Geometry check sheet. Reference: the model listing, model coordinates, mm. A direction names the side the tool comes from. Round coordinates to 2 decimals unless told otherwise and drop trailing zeros. Write each loop counter-clockwise with the first axis right and the second up, starting at its lowest first coordinate (ties: lowest second). Pieces come first, ordered by that corner, then holes. Notation, with made-up numbers: (39.25, 29) - (67.25, 29) arc R33 cw to (67.25, 64) - close; hole circle Ø6 at (20.5, -15.75). An arc over 180 degrees is marked (long way). Return JSON: item names as keys, results as strings.
```python
from build123d import *

# Parameters (mm, degrees)
PAD008_DEPTH = 30
SKETCH003_W  = 24.676034
SKETCH003_H  = 10
PAD002_DEPTH = 25
PAD001_DEPTH = 20
SKETCH002_R  = 5.5
POCKET_DEPTH = 24
PAD007_DEPTH = 40
PAD_DEPTH    = 40


with BuildPart() as pad008:
    # Sketch009 → Pad008 (new body)
    with BuildSketch(Plane.YZ.offset(-17)):
        with BuildLine():
            ThreePointArc((10.172884, 61.128702), (0, 71.301585), (-10.172884, 61.128702))
            Line((-10.172884, 61.128702), (-10.172884, 11.128702))
            ThreePointArc((-10.172884, 11.128702), (0, 0.955818), (10.172884, 11.128702))
            Line((10.172884, 61.128702), (10.172884, 11.128702))
        make_face()
    extrude(amount=PAD008_DEPTH)


with BuildPart() as pad002:
    # Sketch003 → Pad002 (new body)
    with BuildSketch(Plane(origin=(10, 0, 1), x_dir=(1, 0, 0), z_dir=(0, 0, 1))):
        with Locations((25.629245, 0)):
            Rectangle(SKETCH003_W, SKETCH003_H)
    extrude(amount=PAD002_DEPTH)


with BuildPart() as cut:
    # Sketch001 → Pad001 (new body)
    with BuildSketch(Plane(origin=(10, 10, 0), x_dir=(1, 0, 0), z_dir=(0, -1, 0))):
        with BuildLine():
            ThreePointArc((23.375231, 20.790424), (13.375231, 10.790424), (23.375231, 0.790424))
            Line((23.375231, 0.790424), (27.963482, 0.790424))
            ThreePointArc((27.963482, 0.790424), (37.963482, 10.790424), (27.963482, 20.790424))
            Line((23.375231, 20.790424), (27.963482, 20.790424))
        make_face()
    extrude(amount=PAD001_DEPTH)

    # Sketch002 → Pocket (cut)
    with BuildSketch(Plane(origin=(10, -10, 0), x_dir=(1, 0, 0), z_dir=(0, -1, 0))):
        with Locations((25.214981, 10.647934)):
            Circle(SKETCH002_R)
    extrude(amount=-POCKET_DEPTH, mode=Mode.SUBTRACT)

    # Cut: cut Pad002
    add(pad002.part, mode=Mode.SUBTRACT)


with BuildPart() as pad007:
    # Sketch008 → Pad007 (new body)
    with BuildSketch(Plane.XZ.offset(-20)):
        with BuildLine():
            ThreePointArc((11.056906, 25.953392), (1.290425, 15.054425), (-2.307496, 0.868989))
            ThreePointArc((1.093916, 25.953392), (-3.737473, 13.835707), (-2.307496, 0.868989))
            Line((1.093916, 25.953392), (11.056906, 25.953392))
        make_face()
    extrude(amount=PAD007_DEPTH)


with BuildPart() as cut001:
    # Sketch → Pad (new body)
    with BuildSketch(Plane.XZ.offset(-20)):
        with BuildLine():
            Line((-4.143037, -1.678632), (67.891418, -1.678632))
            Line((63.009144, 0.821368), (67.891418, -1.678632))
            Line((-2.143037, 0.821368), (63.009144, 0.821368))
            ThreePointArc((1, 34), (-4.119497, 17.746787), (-2.143037, 0.821368))
            Line((-1, 34), (1, 34))
            ThreePointArc((-1, 34), (-7.73146, 16.615239), (-4.143037, -1.678632))
        make_face()
    extrude(amount=PAD_DEPTH)

    # Fusion001: union Cut, Pad007
    add(cut.part)
    add(pad007.part)

    # Cut001: cut Pad008
    add(pad008.part, mode=Mode.SUBTRACT)


solid = cut001.part
```
(1) Section check B-B, the plane x = 27. Enter the section's corners in (y, z), plus the area to 3 significant figures.
Response values:
{"outline": "(-20, -1.68) - (20, -1.68) - (20, 0.82) - (-20, 0.82) - close; (-10, 3.09) - (-5, 3.09) - (-5, 18.49) - (-10, 18.49) - close; (5, 3.09) - (10, 3.09) - (10, 18.49) - (5, 18.49) - close", "area": "254 mm^2"}
(2) Section check D-D, the plane y = 0. Enter the section's corners in (x, z), plus the area to 3 significant figures.
Response values:
{"outline": "(-5.36, 0.96) arc R33.55 ccw to (-4.14, -1.68) - (67.89, -1.68) - (63.01, 0.82) - (38.75, 0.82) arc R10 ccw to (40, 1) - (31.34, 1) arc R10 ccw to (32.59, 0.82) - (-2.14, 0.82) arc R40.74 cw to (-2.19, 0.96) - close", "area": "177 mm^2"}
(3) Gauge pin test, flat ends, axial feed: pin 1 (2 mm diameter, centred on y = 6.5, z = 20, fed in from -X); pin 2 (16 mm diameter, centred on x = 30, z = 15, fed in from -Y); pin 3 (1.4 mm diameter, centred on x = 36, y = -7, fed in from +Z). Record the tip position at first contact, or that the pin passes through.
Response values:
{"pin 1": "stops at x = 27.67", "pin 2": "stops at y = -10", "pin 3": "stops at z = 20.79"}
(4) Section check A-A, the plane y = 13. Enter the section's corners in (x, z), plus the area to 3 significant figures.
Response values:
{"outline": "(-4.14, -1.68) - (67.89, -1.68) - (63.01, 0.82) - (-2.14, 0.82) arc R40.74 cw to (-2.3, 1.3) arc R30.64 cw to (11.06, 25.95) - (1.09, 25.95) arc R26.93 ccw to (-3.91, 8.3) arc R40.74 cw to (1, 34) - (-1, 34) arc R33.55 ccw to start", "area": "393 mm^2"}
(5) Section check C-C, the plane x = 53. Enter the section's corners in (y, z).
Response values:
{"outline": "(-20, -1.68) - (20, -1.68) - (20, 0.82) - (-20, 0.82) - close"}
(6) Access from +Z, -Z, +X, -X, +Y, -Y to the whole of each face (thin tool, end or side, straight path). Record for faces 5 (the face through (2, 10.173, 20)), 6 (the face through (36, -7, 20.79)), 7 (the face through (6, 15, 25.953)).
Response values:
{"face 5": "+Z, +X, -X", "face 6": "+Z, +X, -X, +Y, -Y", "face 7": "+Z, +X, +Y, -Y"}
(7) Material ranges on line 1 along Y through (x, z) = (0, 17.5); line 2 along Y through (x, z) = (27, 8.5); line 3 along Z through (x, y) = (56.5, -17.5), recorded low to high. Write a range as [from, to].
Response values:
{"line 1": "y = [-20, -10.17], [10.17, 20]", "line 2": "y = [-10, -5], [5, 10]", "line 3": "z = [-1.68, 0.82]"}
(8) Release check for a two-part mould opening along Y. For faces 1 (the face through (-4.16, -0.22, 0.96)), 2 (the face through (41, 10, 11)), 3 (the face through (2, -10.173, 20)), 4 (the face through (65.416, 0.28, -0.411)) record: pulls with the +Y half, pulls with the -Y half, needs draft (parallel to the pull), parting line crosses it, or undercut.
Response values:
{"face 1": "undercut", "face 2": "pulls with the +Y half", "face 3": "undercut", "face 4": "needs draft"}
